Could you check a few things on this drawing? It's one solid part, dimensions in mm from its lowest x, y, z. Give positions to 0.01 mm unless a question says otherwise; leave off trailing zeros. Loops run counter-clockwise (first coordinate to the right, second up) from the corner with the lowest first, then second, coordinate; pieces in that order, holes last. Notation, with made-up numbers: (-32, 58) - (10, 58) arc R17 cw to (10, 67) - close; hole circle Ø10 at (17, 8.25). An arc over 180 degrees is marked (long way). Use a Markdown table: item, result.
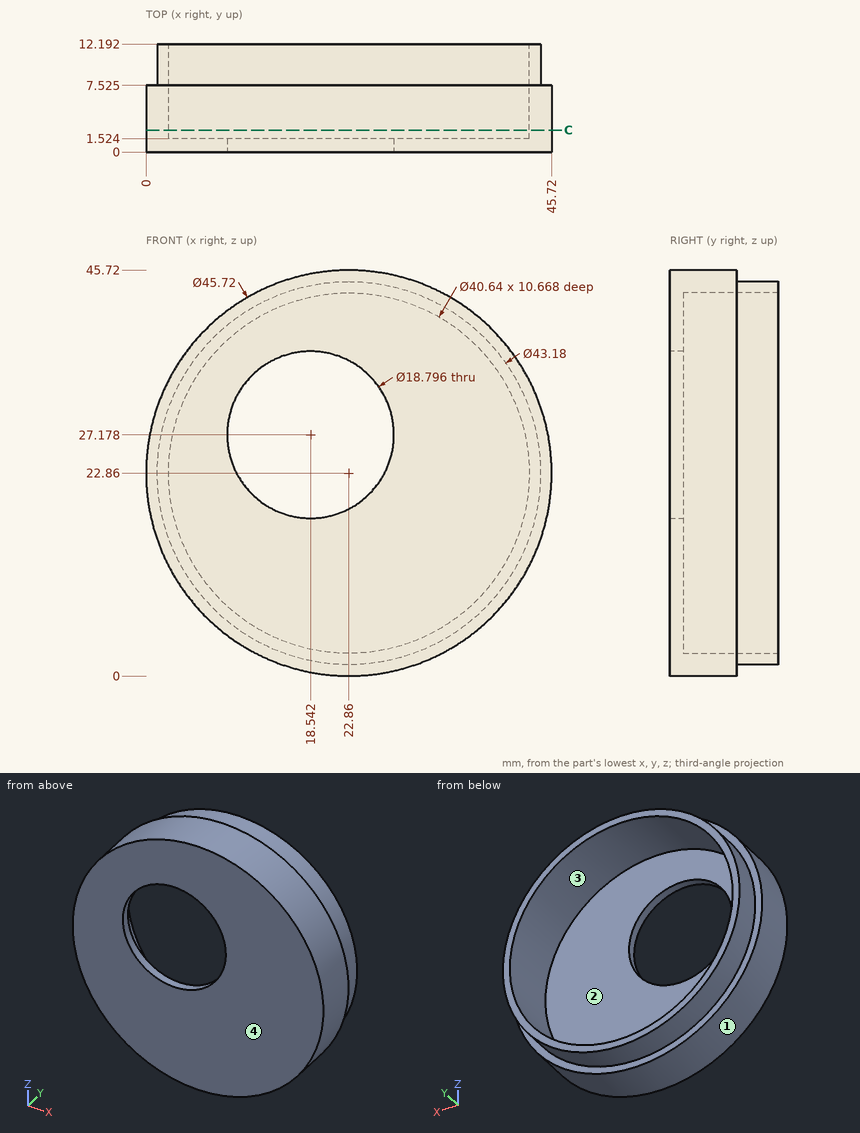
(1) If I drill on line 1 (X direction, y = 7, z = 22.86); line 2 (Z direction, x = 40, y = 9.75) (1 decimal); line 3 (Z direction, x = 35, y = 11) (1 decimal), over which ranges is the centre line in solid material (lowest first)?
A:
| item | result |
|---|---|
| line 1 | 0 to 2.54, 43.18 to 45.72 |
| line 2 | 9.7 to 11.9, 33.8 to 36 |
| line 3 | 5 to 6.6, 39.2 to 40.7 |
(2) Suppose I cut it at C-C on y = 2.5. Write out the boundary of the cut face in (x, z).
A:
| item | result |
|---|---|
| outline | circle Ø45.72 at (22.86, 22.86); hole circle Ø40.64 at (22.86, 22.86) |
(3) Will these pins go through, and if not, where does the flat tip stop? pin 1 (10 mm diameter, centred on x = 17.5, z = 5.5, fed in from +Y); pin 2 (1 mm diameter, centred on x = 38, y = 7.5, fed in from -Z); pin 3 (8 mm diameter, centred on x = 31, z = 17.5, fed in from +Y); pin 4 (5 mm diameter, centred on y = 2, z = 31.5, fed in from +X).
A:
| item | result |
|---|---|
| pin 1 | y = 12.19 |
| pin 2 | z = 5.3 |
| pin 3 | y = 1.52 |
| pin 4 | x = 44.88 |
(4) We'd pull the mould along X, two halves only. Please class the marked faces 1, 2, 3 and 4: pulls with the +X half, pulls with the -X half, needs draft (parallel to the pull), parting line crosses it, or undercut.
A:
| item | result |
|---|---|
| face 1 | parting line crosses it |
| face 2 | undercut |
| face 3 | undercut |
| face 4 | needs draft |
